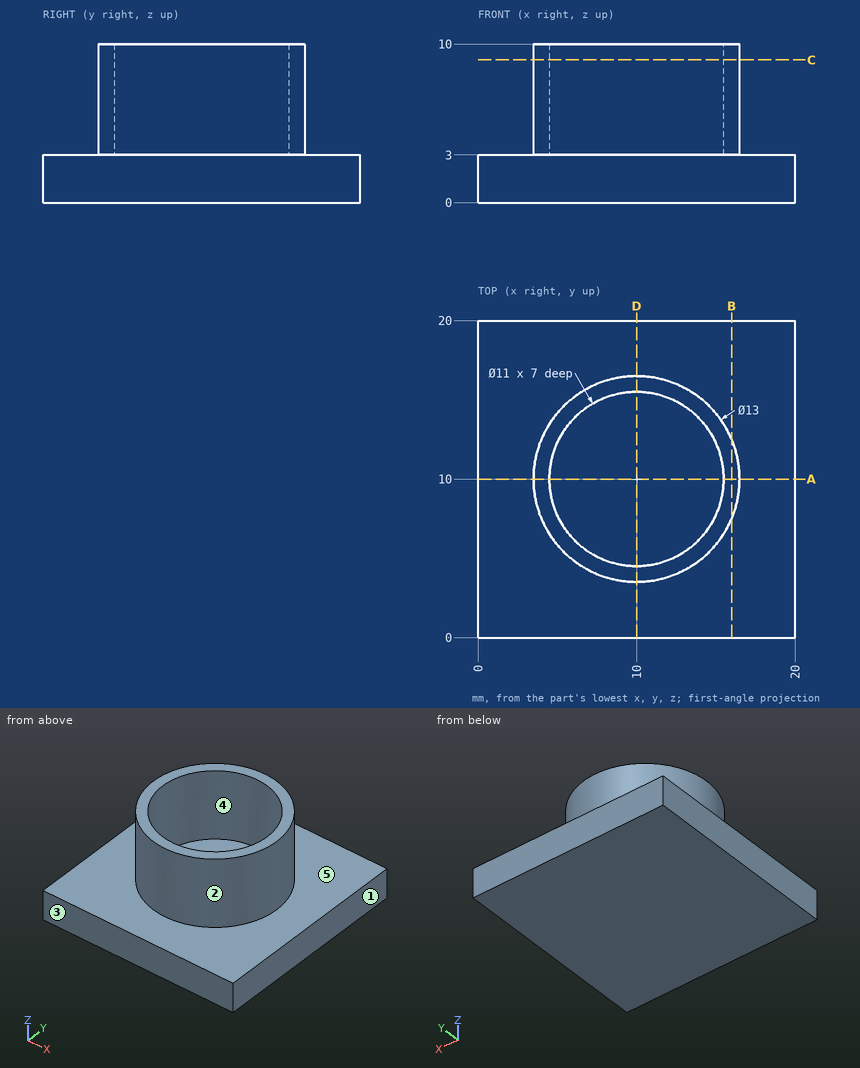
Answer from the drawing. Dimensions are ordinates in mm from the lowest x, y and z of the part. A direction names the side the tool comes from. Round coordinates to 2 decimals unless told otherwise and drop trailing zeros. Write each loop counter-clockwise with the first axis right and the second up, starting at its lowest first coordinate (ties: lowest second). Pieces come first, ordered by that corner, then holes. Notation, with made-up numbers: M 43.25,9 L 91.25,9 A17 cw 91.25,17 Z; hole C 76,-12 d11. An arc over 180 degrees is marked long. Write each question's results on one line, items separated by ' | '. Start each with the question number.
Item 1: The mould has two halves that part along Y. Classify the marked faces 3, 4 and 5: +Y half, -Y half, draft (parallel to the pull), parting line (faces both ways), or undercut.
Item 2: Given pin 1 Ø1.5 at (x, z) = (16, 5) entering from -Y; pin 2 Ø3.5 at (x, y) = (12, 9) entering from +Z; pin 3 Ø4 at (x, z) = (12, 7) entering from -Y, each flat-ended and moving along its own axis, determine where each tip first touches the part or whether it passes through.
Item 3: Find section B-B on x = 16. Write down the section's boundary in (y, z), and give its area (3 significant figures).
Item 4: Find section C-C on z = 9. Write down the section's boundary in (x, y).
Item 5: Which of the six approach directions +Z, -Z, +X, -X, +Y, -Y give full straight-line access (tool end or side, diameter ignored) to the marked faces 1 and 2?
Item 6: Straight lines are drawn through the part: probe 1 along X at (y, z) = (10, 8); probe 2 along Z at (x, y) = (19.25, 2.75). For each, find the intervals that lie inside material, in ascending order.
Item 7: Find section A-A on y = 10. Write down the section's boundary in (x, z), and give its area (3 significant figures).
Answer block:
1) face 3: -Y half | face 4: undercut | face 5: draft
2) pin 1: stops at y = 6.17 | pin 2: stops at z = 3 | pin 3: stops at y = 3.5
3) outline: M 0,0 L 20,0 L 20,3 L 12.5,3 L 12.5,10 L 7.5,10 L 7.5,3 L 0,3 Z | area: 95.0 mm²
4) outline: C 10,10 d13; hole C 10,10 d11
5) face 1: +Z, -Z, +X, +Y, -Y | face 2: +Z
6) probe 1: x = 3.5 to 4.5, 15.5 to 16.5 | probe 2: z = 0 to 3
7) outline: M 0,0 L 20,0 L 20,3 L 16.5,3 L 16.5,10 L 15.5,10 L 15.5,3 L 4.5,3 L 4.5,10 L 3.5,10 L 3.5,3 L 0,3 Z | area: 74.0 mm²
